Geometry: see drawing. Coordinates: mm, zero at the bounding-box minimum. A direction names the side the tool comes from. Coordinates: 2 decimals unless noted, no trailing zeros. Loops run counter-clockwise (first coordinate to the right, second up) from the corner with the lowest first, then second, coordinate; pieces in that order, holes last. Notation, with made-up numbers: (-24.5, 65.25) - (-3.5, 65.25) arc R8 cw to (-3.5, 80.25) - close; hole circle Ø1 at (15.5, 3.25). An arc over 180 degrees is marked (long way). Use one line per item in the form item = value.
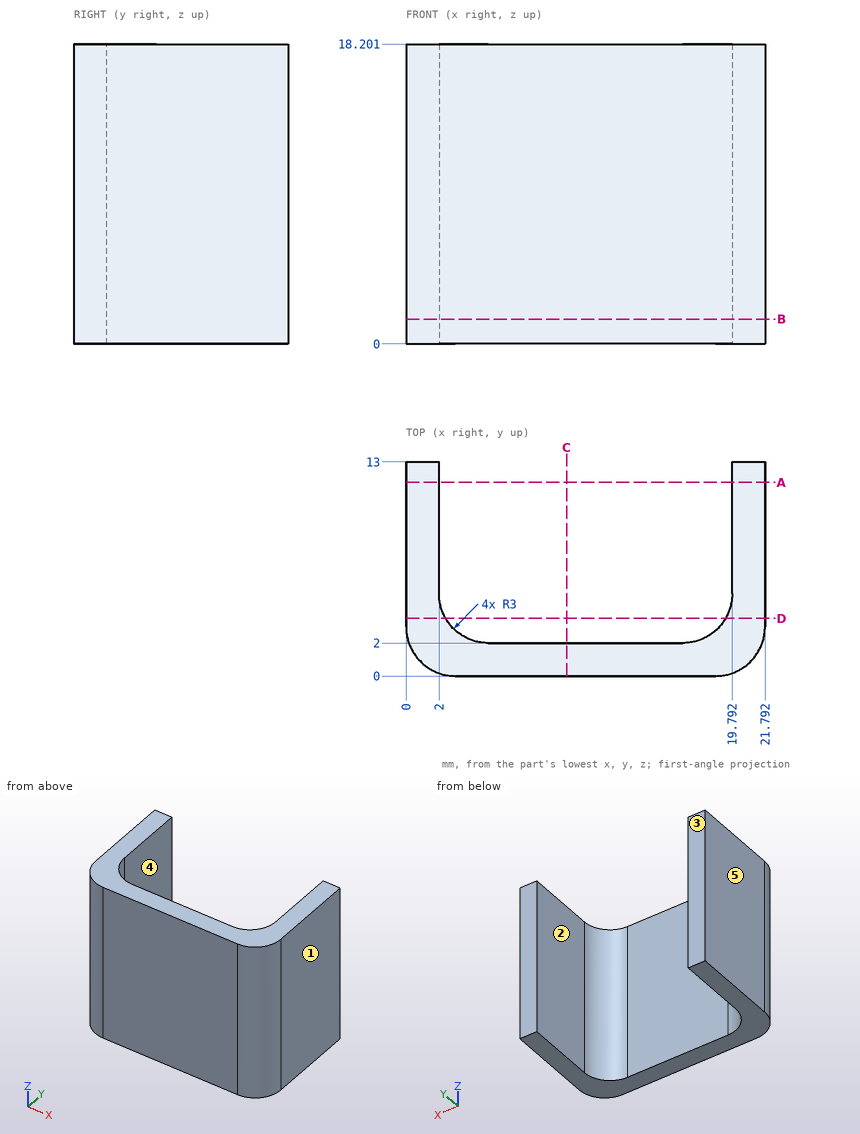
Q1. Cut plane B-B, the plane z = 1.5. Return loops of the section in (x, y).
Check values:
outline = (0, 3) arc R3 ccw to (3, 0) - (18.79, 0) arc R3 ccw to (21.79, 3) - (21.79, 13) - (19.79, 13) - (19.79, 5) arc R3 cw to (16.79, 2) - (5, 2) arc R3 cw to (2, 5) - (2, 13) - (0, 13) - close
Q2. First-contact query: P1, Ø1, axis at x = 17.5, z = 3.5, coming from the +Y side; P2, Ø6, axis at x = 7, y = 11, coming from the +Z side. Flat tips, straight axial feed; report the tip coordinate or a pass-through.
Check values:
P1 = 2.25
P2 = through
Q3. Set-up query: the marked faces 1 and 2. Return all of +Z, -Z, +X, -X, +Y, -Y with unobstructed straight access to the full face (end or side cutting, diameter ignored); none if empty.
Check values:
face_1 = +Z, -Z, +X, +Y, -Y
face_2 = +Z, -Z, +Y
Q4. Cut plane A-A, the plane y = 11.75. Return loops of the section in (x, z).
Check values:
outline = (0, 0) - (2, 0) - (2, 18.2) - (0, 18.2) - close; (19.79, 0) - (21.79, 0) - (21.79, 18.2) - (19.79, 18.2) - close
Q5. Cut plane D-D, the plane y = 3.5. Return loops of the section in (x, z).
Check values:
outline = (0, 0) - (2.4, 0) - (2.4, 18.2) - (0, 18.2) - close; (19.39, 0) - (21.79, 0) - (21.79, 18.2) - (19.39, 18.2) - close
Q6. Cut plane C-C, the plane x = 9.75. Return loops of the section in (y, z).
Check values:
outline = (0, 0) - (2, 0) - (2, 18.2) - (0, 18.2) - close
Q7. Ray query, line 1 along X through (y, z) = (9.25, 9.25); line 2 along Y through (x, z) = (13.75, 3.5); line 3 along X through (y, z) = (4, 6). Return the intervals inside material, ascending. Write a range as [from, to].
Check values:
line_1 = [0, 2], [19.79, 21.79]
line_2 = [0, 2]
line_3 = [0, 2.17], [19.62, 21.79]
Q8. Pull-direction query (X, two-part tool) for the marked faces 3, 4 and 5; classes: pulls with the +X half, pulls with the -X half, needs draft (parallel to the pull), parting line crosses it, or undercut.
Check values:
face_3 = needs draft
face_4 = undercut
face_5 = pulls with the -X half
